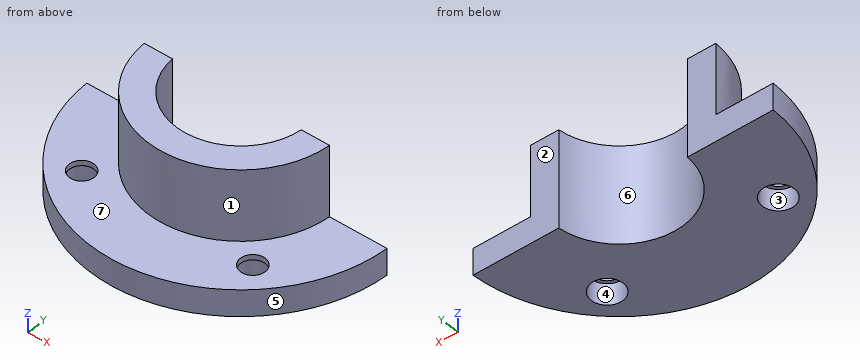
from build123d import *

# Parameters (mm, degrees)
SKETCH1_R               = 85
BOSS_EXTRUDE1_DEPTH     = 15
SKETCH2_R               = 52.5
BOSS_EXTRUDE2_DEPTH     = 40
CUT_EXTRUDE1_DEPTH      = 133.193040664
CUT_EXTRUDE1_DEPTH_BACK = 133.193040664
SKETCH3_R               = 36.5
CUT_EXTRUDE2_DEPTH      = 133.193040664
CUT_EXTRUDE2_DEPTH_BACK = 133.193040664
SKETCH4_W               = 179.422325272
SKETCH4_H               = 89.951571234
CUT_EXTRUDE3_DEPTH      = 133.193040664
CUT_EXTRUDE3_DEPTH_BACK = 133.193040664
SKETCH5_W               = 208.750471757
SKETCH5_H               = 2.5
CUT_EXTRUDE4_DEPTH      = 127.663925409
CUT_EXTRUDE4_DEPTH_BACK = 127.663925409
SKETCH6_R               = 7
SKETCH8_R               = 9
CUT_EXTRUDE5_DEPTH      = 12


with BuildPart() as part:
    # Sketch1 → Boss-Extrude1 (new body)
    with BuildSketch(Plane.XY):
        Circle(SKETCH1_R)
    extrude(amount=BOSS_EXTRUDE1_DEPTH)

    # Sketch2 → Boss-Extrude2 (add)
    with BuildSketch(Plane.XY.offset(15)):
        Circle(SKETCH2_R)
    extrude(amount=BOSS_EXTRUDE2_DEPTH)

    # Sketch3 → Cut-Extrude1 (cut, two sides: drawn at the far end of the back side and taken through both)
    with BuildSketch(Plane.XY.offset(55).offset(-CUT_EXTRUDE1_DEPTH_BACK)):
        Circle(SKETCH3_R)
    extrude(amount=CUT_EXTRUDE1_DEPTH + CUT_EXTRUDE1_DEPTH_BACK, mode=Mode.SUBTRACT)

    # Sketch4 → Cut-Extrude2 (cut, two sides: drawn at the far end of the back side and taken through both)
    with BuildSketch(Plane.XY.offset(55).offset(-CUT_EXTRUDE2_DEPTH_BACK)):
        with Locations((-4.711162636, 44.975785617)):
            Rectangle(SKETCH4_W, SKETCH4_H)
    extrude(amount=CUT_EXTRUDE2_DEPTH + CUT_EXTRUDE2_DEPTH_BACK, mode=Mode.SUBTRACT)

    # Sketch5 → Cut-Extrude3 (cut, two sides: drawn at the far end of the back side and taken through both)
    with BuildSketch(Plane.XY.offset(55).offset(-CUT_EXTRUDE3_DEPTH_BACK)):
        with Locations((-19.375235879, -1.25)):
            Rectangle(SKETCH5_W, SKETCH5_H)
    extrude(amount=CUT_EXTRUDE3_DEPTH + CUT_EXTRUDE3_DEPTH_BACK, mode=Mode.SUBTRACT)

    # Sketch6 → Cut-Extrude4 (cut, two sides: drawn at the far end of the back side and taken through both)
    with BuildSketch(Plane.XY.offset(15).offset(-CUT_EXTRUDE4_DEPTH_BACK)):
        with Locations((48.436814511, -48.436814511)):
            Circle(SKETCH6_R)
        with Locations((-48.436814511, -48.436814511)):
            Circle(SKETCH6_R)
    extrude(amount=CUT_EXTRUDE4_DEPTH + CUT_EXTRUDE4_DEPTH_BACK, mode=Mode.SUBTRACT)

    # Sketch8 → Cut-Extrude5 (cut)
    with BuildSketch(Plane(origin=(0, 0, 0), x_dir=(-1, 0, 0), z_dir=(0, 0, -1))):
        with Locations((-48.436814511, -48.436814511)):
            Circle(SKETCH8_R)
        with Locations((48.436814511, -48.436814511)):
            Circle(SKETCH8_R)
    extrude(amount=-CUT_EXTRUDE5_DEPTH, mode=Mode.SUBTRACT)


solid = part.part
Input: part model. Units: mm. Frame: model coordinates. Face numbers are marked on the shaded views. A direction names the side the tool comes from. Round coordinates to 2 decimals unless told otherwise and drop trailing zeros. Write each loop counter-clockwise with the first axis right and the second up, starting at its lowest first coordinate (ties: lowest second). Pieces come first, ordered by that corner, then holes.
1) Reachability of the marked faces 1, 2 and 3 from +Z, -Z, +X, -X, +Y, -Y: full face, straight path, thin tool, end or side. Return the list, or none.
2) Cut plane C-C (x = 0). Return the cut outline in (y, z), then the cut area to 3 significant figures.
3) Cut plane D-D (z = 31). Return the cut outline in (x, y).
4) Cut plane A-A (y = -12.5). Return the cut outline in (x, z), then the cut area to 3 significant figures.
5) Contact query for flat-ended pins moving along their axis: P1, Ø16, axis at x = 48.44, y = -48.44, coming from the -Z side; P2, Ø6, axis at x = 34.5, z = 7.5, coming from the -Y side; P3, Ø11, axis at x = -48.44, y = -48.44, coming from the -Z side; P4, Ø6, axis at x = -16, z = 16.5, coming from the +Y side. Output: stop coordinate, or through.
6) Cut plane B-B (x = 50.5). Return the cut outline in (y, z), then the cut area to 3 significant figures.
7) Draft query along Y for the marked faces 4, 5, 6 and 7. Return one class per face: pulls with the +Y half, pulls with the -Y half, needs draft (parallel to the pull), parting line crosses it, or undercut.
8) Ray query, L1, parallel to X at y = -19.5, z = 8; L2, parallel to Y at x = -1, z = 47; L3, parallel to Y at x = -42.5, z = 14. Return the intervals inside material, ascending.
Geometry says:
1. face 1: +Z, -Y
1. face 2: +Z, -Z, +X, -X, +Y
1. face 3: -Z
2. outline: (-85, 0) - (-36.5, 0) - (-36.5, 55) - (-52.5, 55) - (-52.5, 15) - (-85, 15) - close
2. area: 1,370 mm2
3. outline: (-52.44, -2.5) arc R52.5 ccw to (52.44, -2.5) - (36.41, -2.5) arc R36.5 cw to (-36.41, -2.5) - close
4. outline: (-84.08, 0) - (-34.29, 0) - (-34.29, 55) - (-50.99, 55) - (-50.99, 15) - (-84.08, 15) - close; (34.29, 0) - (84.08, 0) - (84.08, 15) - (50.99, 15) - (50.99, 55) - (34.29, 55) - close
4. area: 2,830 mm2
5. P1: stops at z = 12
5. P2: stops at y = -78.95
5. P3: passes through
5. P4: stops at y = -31.16
6. outline: (-68.37, 0) - (-57.2, 0) - (-57.2, 12) - (-55.13, 12) - (-55.13, 15) - (-68.37, 15) - close; (-41.75, 12) - (-39.68, 12) - (-39.68, 0) - (-2.5, 0) - (-2.5, 55) - (-14.35, 55) - (-14.35, 15) - (-41.75, 15) - close
6. area: 1,210 mm2
7. face 4: undercut
7. face 5: pulls with the -Y half
7. face 6: pulls with the +Y half
7. face 7: needs draft
8. L1: x = -82.73 to -30.85, 30.85 to 82.73
8. L2: y = -52.49 to -36.49
8. L3: y = -73.61 to -52.15, -44.73 to -2.5
